Geometry check sheet. Reference: the model listing, model coordinates, mm. Round coordinates to 2 decimals unless told otherwise and drop trailing zeros. Order: outer loops, then holes, each group sorted by start corner. A loop starts at its lowest first (then second) coordinate and runs counter-clockwise, first axis right, second up. Notation, with made-up numbers: (41.25, 4.5) - (89.25, 4.5) arc R33 ccw to (89.25, 35.5) - close; hole circle Ø10 at (31.5, 29.5). An arc over 180 degrees is marked (long way). Return JSON: item names as keys, results as strings. Group by question number.
Q1. Material ranges on line 1 along X through (y, z) = (-33.5, -94); line 2 along X through (y, z) = (-24, 110.5); line 3 along Z through (x, y) = (70, -52.5), recorded low to high.
Q2. Sectioned sample at B-B, the plane z = 21. Record the cut outline in (x, y), then the cut area to 3 significant figures.
Q3. Gauge pin test, flat ends, axial feed: pin 1 Ø1.5 at (y, z) = (-5, -54.5) entering from +X; pin 2 Ø3 at (x, y) = (-125.5, -35) entering from -Z; pin 3 Ø7 at (x, z) = (-3, -1.5) entering from +Y. Record the tip position at first contact, or that the pin passes through.
Q4. Sectioned sample at A-A, the plane y = -2.5. Record the cut outline in (x, z).
Q5. Sectioned sample at C-C, the plane x = -74.5. Record the cut outline in (y, z).
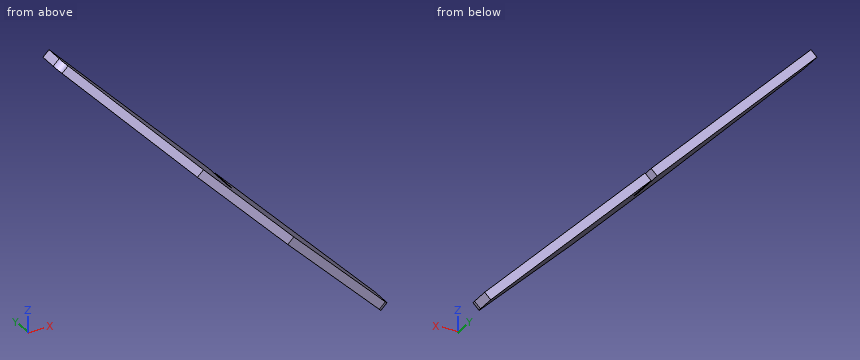
```python
from build123d import *

# Parameters (mm, degrees)
BOSS_EXTRUDE1_DEPTH     = 15
BOSS_EXTRUDE2_DEPTH     = 5
CUT_EXTRUDE2_DEPTH      = 284.32843133
CUT_EXTRUDE2_DEPTH_BACK = 284.32843133
SKETCH4_W               = 10.2
SKETCH4_H               = 82
FILLET1_R               = 10


with BuildPart() as part:
    # Sketch1 → Boss-Extrude1 (new, symmetric)
    with BuildSketch(Plane(origin=(0, 0, 0), x_dir=(1, 0, 0), z_dir=(0, 1, 0))):
        Polygon((-195, -187.928932188), (-187.928932188, -195), (195, 187.928932188), (187.928932188, 195), align=None)
    extrude(amount=BOSS_EXTRUDE1_DEPTH, both=True)

    # Sketch3 → Boss-Extrude2 (add, symmetric)
    with BuildSketch(Plane(origin=(0, 0, 0), x_dir=(0.7071067811865476, 0, -0.7071067811865476), z_dir=(0.7071067811865476, 0, 0.7071067811865476))):
        Polygon((270.771644663, -15), (75, -65), (-75, -65), (-270.771644663, -15), align=None)
    extrude(amount=BOSS_EXTRUDE2_DEPTH, both=True)

    # Sketch4 → Cut-Extrude2 (cut, two sides: drawn at the far end of the back side and taken through both)
    with BuildSketch(Plane(origin=(0, 0, 0), x_dir=(0.7071067811865476, 0, -0.7071067811865476), z_dir=(0.7071067811865476, 0, 0.7071067811865476)).offset(-CUT_EXTRUDE2_DEPTH_BACK)):
        with Locations((-0.430935361, 15)):
            Rectangle(SKETCH4_W, SKETCH4_H)
    extrude(amount=CUT_EXTRUDE2_DEPTH + CUT_EXTRUDE2_DEPTH_BACK, mode=Mode.SUBTRACT)

    # Fillet1
    fillet1_edges = [part.edges().sort_by_distance(p)[0] for p in [
        (191.464466094, -15, -191.464466094),
        (-191.464466094, -15, 191.464466094),
    ]]
    fillet(fillet1_edges, radius=FILLET1_R)


solid = part.part
```
Reply:
{
 "1": {"line 1": "86.93 to 101.07", "line 2": "-117.57 to -103.43", "line 3": "-77.07 to -62.93"},
 "2": {"outline": "(-28.07, -65) - (-13.93, -65) - (-13.93, 15) - (-28.07, 15) - close", "area": "1,130 mm^2"},
 "3": {"pin 1": "x = 62.32", "pin 2": "z = 116.93", "pin 3": "y = -26"},
 "4": {"outline": "(-195, 187.93) - (-7.45, 0.38) - (-0.38, 7.45) - (-187.93, 195) - close; (-0.23, -6.84) - (187.93, -195) - (195, -187.93) - (6.84, 0.23) - close"},
 "5": {"outline": "(-58.52, 67.43) - (15, 67.43) - (15, 81.57) - (-55.97, 81.57) - close"}
}
